from build123d import *

# Parameters (mm, degrees)
DODANIE_WYCI_GNI_CIE1_DEPTH = 5.2
SZKIC3_W                    = 60
SZKIC3_H                    = 159.9
SZKIC5_W                    = 99.9
SZKIC5_H                    = 199.8
SZKIC6_W                    = 49.271239353
SZKIC6_H                    = 120
WYTNIJ_WYCI_GNI_CIE1_DEPTH  = 78
WYTNIJ_WYCI_GNI_CIE2_DEPTH  = 5.6
SZKIC9_R                    = 2.424871131
SZKIC9_R_2                  = 1.2
DODANIE_WYCI_GNI_CIE3_DEPTH = 3.8
SZKIC10_W                   = 50
SZKIC10_H                   = 39.9
WYTNIJ_WYCI_GNI_CIE4_DEPTH  = 24
DODANIE_WYCI_GNI_CIE4_DEPTH = 39.9
DODANIE_WYCI_GNI_CIE5_DEPTH = 45.5


with BuildPart() as part:
    # Szkic2 → Dodanie-wyciągnięcie1 (new body)
    with BuildSketch(Plane.XY):
        Polygon((18.542832418, 83.245366469), (18.542832418, 43.345366469), (-51.457167582, 43.345366469), (-51.457167582, -76.654633531), (18.542832418, -76.654633531), (18.542832418, -116.554633531), (-81.357167582, -116.554633531), (-81.357167582, 83.245366469), align=None)
    extrude(amount=DODANIE_WYCI_GNI_CIE1_DEPTH)

    # Szkic3 → Wyciągnięcie po profilach3 section 0
    with BuildSketch(Plane.XY.offset(11.5)):
        with Locations((-11.457167582, 3.295366469)):
            Rectangle(SZKIC3_W, SZKIC3_H)
    # Szkic5 → Wyciągnięcie po profilach3 section 1
    with BuildSketch(Plane.XY.offset(5.2)):
        with Locations((-31.407167582, -16.654633531)):
            Rectangle(SZKIC5_W, SZKIC5_H)
    loft()

    # Szkic6 → Wytnij-wyciągnięcie1 (cut)
    with BuildSketch(Plane(origin=(-51.457167582, 0, 0), x_dir=(0, 0, -1), z_dir=(1, 0, 0))):
        with Locations((-24.635619677, -16.654633531)):
            Rectangle(SZKIC6_W, SZKIC6_H)
    extrude(amount=WYTNIJ_WYCI_GNI_CIE1_DEPTH, mode=Mode.SUBTRACT)

    # Szkic7 → Wytnij-wyciągnięcie2 (cut)
    with BuildSketch(Plane(origin=(-51.457167582, 0, 0), x_dir=(0, 0, -1), z_dir=(1, 0, 0))):
        Polygon((-5.12, -34.1297624), (-7.22, -35.342197966), (-7.22, -37.767069096), (-5.12, -38.979504662), (-3.02, -37.767069096), (-3.02, -35.342197966), align=None)
        Polygon((-5.12, 5.6702376), (-7.22, 4.457802034), (-7.22, 2.032930904), (-5.12, 0.820495338), (-3.02, 2.032930904), (-3.02, 4.457802034), align=None)
    extrude(amount=-WYTNIJ_WYCI_GNI_CIE2_DEPTH, mode=Mode.SUBTRACT)

    # Szkic9 → Dodanie-wyciągnięcie3 (add)
    with BuildSketch(Plane(origin=(-51.457167582, 0, 0), x_dir=(0, 0, -1), z_dir=(1, 0, 0))):
        with Locations((-5.12, 3.245366469)):
            Circle(SZKIC9_R)
        with Locations((-5.12, 3.245366469)):
            Circle(SZKIC9_R_2, mode=Mode.SUBTRACT)
        with Locations((-5.12, -36.554633531)):
            Circle(SZKIC9_R)
        with Locations((-5.12, -36.554633531)):
            Circle(SZKIC9_R_2, mode=Mode.SUBTRACT)
    extrude(amount=-DODANIE_WYCI_GNI_CIE3_DEPTH)

    # Szkic10 → Wytnij-wyciągnięcie4 (cut)
    with BuildSketch(Plane.XY.offset(11.5)):
        with Locations((-6.457167582, 63.295366469)):
            Rectangle(SZKIC10_W, SZKIC10_H)
    extrude(amount=-WYTNIJ_WYCI_GNI_CIE4_DEPTH, mode=Mode.SUBTRACT)

    # Szkic12 → Dodanie-wyciągnięcie4 (add)
    with BuildSketch(Plane(origin=(0, 83.245366469, 0), x_dir=(1, 0, 0), z_dir=(0, 1, 0))):
        Polygon((-31.457167582, -11.5), (-26.957167582, -11.5), (-26.957167582, -10.5), (-31.457167582, -8), align=None)
    extrude(amount=-DODANIE_WYCI_GNI_CIE4_DEPTH)

    # Szkic13 → Dodanie-wyciągnięcie5 (add)
    with BuildSketch(Plane(origin=(18.542832418, 0, 0), x_dir=(0, 0, -1), z_dir=(1, 0, 0))):
        Polygon((-11.5, -76.654633531), (-1.5, -76.654633531), (-10.5, -66.654633531), (-11.5, -66.654633531), align=None)
    extrude(amount=-DODANIE_WYCI_GNI_CIE5_DEPTH)


solid = part.part
The listing builds one solid part. Answer for the finished solid, in the listing's coordinates (mm). A direction names the side the tool comes from. Give positions to 0.01 mm unless a question says otherwise; leave off trailing zeros.
1) Given P1, Ø6, axis at y = 4, z = 6, coming from the +X side; P2, Ø2, axis at y = -36.55, z = 5.12, coming from the +X side; P3, Ø6, axis at x = -40.5, z = 7, coming from the -Y side; P4, Ø1.1, axis at y = 73, z = 11, coming from the +X side, each flat-ended and moving along its own axis, determine where each tip first touches the part or whether it passes through.
2) For a pull along Y with two mould halves and no side action, classify faces 6 (the face through (-55, 83.245, 4)), 7 (the face through (-42, 43.345, 6)), 8 (the face through (-53, -37, 0)) as pulls with the +Y half, pulls with the -Y half, needs draft (parallel to the pull), parting line crosses it, or undercut.
3) Find the intervals of material crossed by L1, parallel to Y at x = -52.7, z = 5.12; L2, parallel to X at y = 62, z = 1; L3, parallel to X at y = 36, z = 3, in increasing order.
4) A tool of negligible diameter and unlimited length cuts with its end or side. For faces 1 (the face through (-31, -116.555, 3)), 2 (the face through (-33, -76.655, 5)), 3 (the face through (-57.057, 3, 5)), 4 (the face through (-26.957, -73, 8)), 5 (the face through (-31.457, 63, 4)), from which of +Z, -Z, +X, -X, +Y, -Y can it reach the whole face along a straight path? Write none if from no direction.
Response:
1. P1: stops at x = -51.46
1. P2: stops at x = -57.06
1. P3: stops at y = -116.55
1. P4: stops at x = -26.96
2. face 6: pulls with the +Y half
2. face 7: undercut
2. face 8: needs draft
3. L1: y = -116.55 to -37.75, -35.35 to 2.05, 4.45 to 83.25
3. L2: x = -81.36 to -31.46
3. L3: x = -81.36 to -51.46
4. face 1: +Z, -Z, +X, -X, -Y
4. face 2: -Z
4. face 3: none
4. face 4: +Z, -Z
4. face 5: -Z, +X, +Y
